```python
from build123d import *

# Parameters (mm, degrees)
SKETCH1_R           = 2.50825
BOSS_EXTRUDE1_DEPTH = 10
FILLET1_R           = 3.175
CHAMFER1_SIZE       = 3.175


with BuildPart() as part:
    # Sketch1 → Boss-Extrude1 (new body)
    with BuildSketch(Plane(origin=(0, 0, 0), x_dir=(1, 0, 0), z_dir=(0, 1, 0))):
        with BuildLine():
            Line((0, 30), (0, 0))
            Line((0, 0), (42.5, 0))
            ThreePointArc((42.5, 0), (50, 7.5), (42.5, 15))
            Line((42.5, 15), (15.875, 15))
            Line((15.875, 15), (15.875, 30))
            Line((15.875, 30), (0, 30))
        make_face()
        with Locations((7.9375, 23.175)):
            Circle(SKETCH1_R, mode=Mode.SUBTRACT)
    extrude(amount=BOSS_EXTRUDE1_DEPTH)

    # Fillet1
    fillet1_edges = [part.edges().sort_by_distance(p)[0] for p in [
        (0, 5, 0),
    ]]
    fillet(fillet1_edges, radius=FILLET1_R)

    # Chamfer1
    chamfer1_edges = [part.edges().sort_by_distance(p)[0] for p in [
        (15.875, 5, -30),
        (0, 5, -30),
    ]]
    chamfer(chamfer1_edges, length=CHAMFER1_SIZE)


solid = part.part
```
The model under review builds one solid part; all positions refer to its coordinate system, in mm. A direction names the side the tool comes from. Coordinates: 2 decimals unless noted, no trailing zeros. Write each loop counter-clockwise with the first axis right and the second up, starting at its lowest first coordinate (ties: lowest second). Pieces come first, ordered by that corner, then holes. Notation, with made-up numbers: (40, 73) -> (57, 73) arc R7 cw to (57, 83) -> close; hole circle Ø9 at (80.25, 3.5). An arc over 180 degrees is marked (long way). One line per item, written item: value. Start each with the question number.
Q1. Clearance check with flat-ended pins moving along their axes: P1, Ø1.5, axis at x = 19, y = 8.5, coming from the -Z side; P2, Ø4, axis at y = 6.5, z = -25, coming from the +X side (3 decimals). State where each tip first meets the part, or that it passes through.
Q2. To check wall thickness, follow probe 1 along Z at (x, y) = (18, 7); probe 2 along X at (y, z) = (4, -22.5) (3 decimals); probe 3 along X at (y, z) = (6, -18) (3 decimals). State the ranges of each line that lie inside material, in increasing order.
Q3. Add section B-B, the plane x = 7. Give the boundary of the cut face in (y, z).
Q4. Add section D-D, the plane x = 39. Give the boundary of the cut face in (y, z).
Q5. The part is to be moulded in two halves that separate along Z. For faces 1 (the face through (7.394, 4.93, -20.726)), 2 (the face through (23, 5, 0)), 3 (the face through (8, 5, -30)), 4 (the face through (50, 4.93, -7.34)), say which applies: +Z half, -Z half, draft (parallel to the pull), parting line (faces both ways), or undercut.
Q6. For faces 5 (the face through (19, 0, -12)), 6 (the face through (29, 5, -15)), list the 3-axis set-ups (+Z, -Z, +X, -X, +Y, -Y) from which the entire face can be reached by the end or side of a thin tool; tool diameter is ignored.
Q7. Add section A-A, the plane z = -25. Give the boundary of the cut face in (x, y) (3 decimals), then the cut area to 3 significant figures.
Response:
1. P1: z = -15
1. P2: x = 15.875
2. probe 1: -15 to 0
2. probe 2: 0 to 5.522, 10.353 to 15.875
2. probe 3: 0 to 15.875
3. outline: (0, -30) -> (10, -30) -> (10, -25.5) -> (0, -25.5) -> close; (0, -20.85) -> (10, -20.85) -> (10, 0) -> (0, 0) -> close
4. outline: (0, -15) -> (10, -15) -> (10, 0) -> (0, 0) -> close
5. face 1: undercut
5. face 2: +Z half
5. face 3: -Z half
5. face 4: parting line
6. face 5: +Z, -Z, +X, -X, -Y
6. face 6: -Z, +X, +Y, -Y
7. outline: (0, 0) -> (6.217, 0) -> (6.217, 10) -> (0, 10) -> close; (9.658, 0) -> (15.875, 0) -> (15.875, 10) -> (9.658, 10) -> close
7. area: 124 mm²
